```python
from build123d import *

# Parameters (mm, degrees)
AUFSATZ_LINEAR_AUSTRAGEN1_DEPTH = 15
SKIZZE8_W                       = 15
SKIZZE8_H                       = 1.8
AUFSATZ_LINEAR_AUSTRAGEN2_DEPTH = 3.6
SKIZZE9_W                       = 1.8
SKIZZE9_H                       = 15
AUFSATZ_LINEAR_AUSTRAGEN3_DEPTH = 1.8
SKIZZE10_W                      = 1.8
SKIZZE10_H                      = 15
AUFSATZ_LINEAR_AUSTRAGEN4_DEPTH = 1.8


# Read off the part's stored shape, not the designer's step: Aufsatz-Linear austragen1
with BuildPart() as part:
    # Aufsatz-Linear austragen1 outline → Aufsatz-Linear austragen1 (new body)
    with BuildSketch(Plane.XY):
        with BuildLine():
            Line((7, 7.5), (7, 5.522993755))
            add(Edge.make_bspline(
                [(7, 5.522993755), (0.965861159, -1.223721572), (4, -9.5)],
                knots=[0.129703712, 0.129703712, 0.129703712, 1, 1, 1], degree=2))
            Line((4, -9.5), (4.938894523, -9.155795009))
            add(Edge.make_bspline(
                [(9, 6.145084082), (8.894106899, 6.044673778), (8.472209731, 5.637376992), (7.500876339, 4.623469608), (6.267154764, 3.067786271), (5.159309564, 1.168794415), (4.408096908, -0.769290789), (4.005150376, -2.755259304), (3.945419318, -4.803083613), (4.18652921, -6.57746866), (4.554595844, -8.031875726), (4.803987208, -8.787813624), (4.938894523, -9.155795009)],
                knots=[0.041945828, 0.041945828, 0.041945828, 0.041945828, 0.0625, 0.125, 0.25, 0.375, 0.5, 0.625, 0.75, 0.875, 0.9375, 1, 1, 1, 1], degree=3))
            Line((9, 6.145084082), (9, 9.5))
            Line((9, 9.5), (-1, 9.5))
            Line((-1, 9.5), (-1, -9.5))
            Line((-1, -9.5), (1, -9.5))
            Line((1, -9.5), (1, 7.5))
            Line((1, 7.5), (7, 7.5))
        make_face()
    extrude(amount=AUFSATZ_LINEAR_AUSTRAGEN1_DEPTH)

    # Skizze8 → Aufsatz-Linear austragen2 (add)
    with BuildSketch(Plane.ZY.offset(1)):
        with Locations((7.5, 8.6)):
            Rectangle(SKIZZE8_W, SKIZZE8_H)
        with Locations((7.5, -8.6)):
            Rectangle(SKIZZE8_W, SKIZZE8_H)
    extrude(amount=AUFSATZ_LINEAR_AUSTRAGEN2_DEPTH)

    # Skizze9 → Aufsatz-Linear austragen3 (add)
    with BuildSketch(Plane(origin=(0, -7.7, 0), x_dir=(1, 0, 0), z_dir=(0, 1, 0))):
        with Locations((-3.7, -7.5)):
            Rectangle(SKIZZE9_W, SKIZZE9_H)
    extrude(amount=AUFSATZ_LINEAR_AUSTRAGEN3_DEPTH)

    # Skizze10 → Aufsatz-Linear austragen4 (add)
    with BuildSketch(Plane.XZ.offset(-7.7)):
        with Locations((-3.7, 7.5)):
            Rectangle(SKIZZE10_W, SKIZZE10_H)
    extrude(amount=AUFSATZ_LINEAR_AUSTRAGEN4_DEPTH)


solid = part.part
```
Build history of the part. All positions in model axes, mm. A direction names the side the tool comes from. Coordinates: 2 decimals unless noted, no trailing zeros. Order: outer loops, then holes, each group sorted by start corner. A loop starts at its lowest first (then second) coordinate and runs counter-clockwise, first axis right, second up. Notation, with made-up numbers: (61, 79) -> (87, 79) arc R21 cw to (87, 89) -> close; hole circle Ø11 at (-40, -19.75). An arc over 180 degrees is marked (long way). Answer in a Markdown table with one row per item. Add a question column.
Q1. Which spindle directions (+Z, -Z, +X, -X, +Y, -Y) get a long thin tool onto all of the face, cutting with end or side? Do faces 1 (the face through (-2, 7.7, 7)), 2 (the face through (1, -1, 7)), 3 (the face through (-4, -5.9, 7)). Say none if no direction does.
Q2. Mould opens along Y. For faces 4 (the face through (4.46, -9.33, 7.4)), 5 (the face through (7, 7, 7)), 6 (the face through (2, 9.5, 7)), 7 (the face through (9, 8, 7)) say: +Y half, -Y half, draft (parallel to the pull), parting line (faces both ways), or undercut.
Q3. Drop flat-ended pins along their axis: pin 1 (0.9 mm diameter, centred on y = -7, z = 11, fed in from +X); pin 2 (7.5 mm diameter, centred on y = -2, z = 4, fed in from +X); pin 3 (4 mm diameter, centred on x = 3, z = 7, fed in from -Y); pin 4 (3 mm diameter, centred on x = -3, y = 6.5, fed in from -Z). Give the stop position or say it passes through.
Q4. Band-saw the part on A-A, the plane x = -2.5. List the corners of the cut face in (y, z).
Q5. Band-saw the part on B-B, the plane x = 2.25. List the corners of the cut face in (y, z), then the cut area to 3 significant figures.
Q6. Wall check: line 1 along X through (y, z) = (-4, 2.5); line 2 along Y through (x, z) = (-2.75, 3); line 3 along Y through (x, z) = (-3.25, 14.5). Give the ranges that are in metal, low to high. Write a range as [from, to].
Answers follow:
| question | item | result |
|---|---|---|
| 1 | face 1 | +Z, -Z |
| 1 | face 2 | +Z, -Z, -Y |
| 1 | face 3 | +Z, -Z, -X |
| 2 | face 4 | -Y half |
| 2 | face 5 | undercut |
| 2 | face 6 | +Y half |
| 2 | face 7 | draft |
| 3 | pin 1 | x = 4.41 |
| 3 | pin 2 | x = 5.52 |
| 3 | pin 3 | y = -9.5 |
| 3 | pin 4 | z = 0 |
| 4 | outline | (-9.5, 0) -> (-7.7, 0) -> (-7.7, 15) -> (-9.5, 15) -> close; (7.7, 0) -> (9.5, 0) -> (9.5, 15) -> (7.7, 15) -> close |
| 5 | outline | (7.5, 0) -> (9.5, 0) -> (9.5, 15) -> (7.5, 15) -> close |
| 5 | area | 30.0 mm^2 |
| 6 | line 1 | [-1, 1], [2.99, 3.99] |
| 6 | line 2 | [-9.5, -7.7], [7.7, 9.5] |
| 6 | line 3 | [-9.5, -5.9], [5.9, 9.5] |
